Geometry: see drawing. Coordinates: mm, zero at the bounding-box minimum. A direction names the side the tool comes from. Coordinates: 2 decimals unless noted, no trailing zeros. Loops run counter-clockwise (first coordinate to the right, second up) from the corner with the lowest first, then second, coordinate; pieces in that order, holes last. Notation, with made-up numbers: M 47,83.5 L 98,83.5 A19 cw 98,104.5 Z; hole C 10,-23.5 d8. An arc over 180 degrees is marked long. One line per question, with ' | ' between items. Start each with the question number.
1. Ray query, probe 1 along Z at (x, y) = (2.5, 10); probe 2 along Y at (x, z) = (1.5, 5); probe 3 along Y at (x, z) = (8, 7.25). Return the intervals inside material, ascending.
2. Section query C-C, the plane x = 2. Output: boundary loops of the cut face in (y, z), and give its area (3 significant figures).
3. Section query A-A, the plane z = 11.5. Output: boundary loops of the cut face in (x, y), and give its area (3 significant figures).
4. Pin query (flat end, axial travel): P1, Ø1, axis at x = 7, y = 27, coming from the +Z side. Return the tip coordinate at first contact, or that it passes through.
5. Access query for the marked faces 1 and 2. Directions: +Z, -Z, +X, -X, +Y, -Y. A direction counts if a zero-diameter tool reaches every point of the face in a straight line with its end or side. Return the directions, or none.
6. Section query D-D, the plane z = 3.5. Output: boundary loops of the cut face in (x, y), and give its area (3 significant figures).
7. Mould query, pull axis Z, two halves, no side actions, for the marked faces 3, 4 and 5. Classes: pulls with the +Z half, pulls with the -Z half, needs draft (parallel to the pull), parting line crosses it, or undercut.
8. Section query B-B, the plane y = 10. Output: boundary loops of the cut face in (x, z).
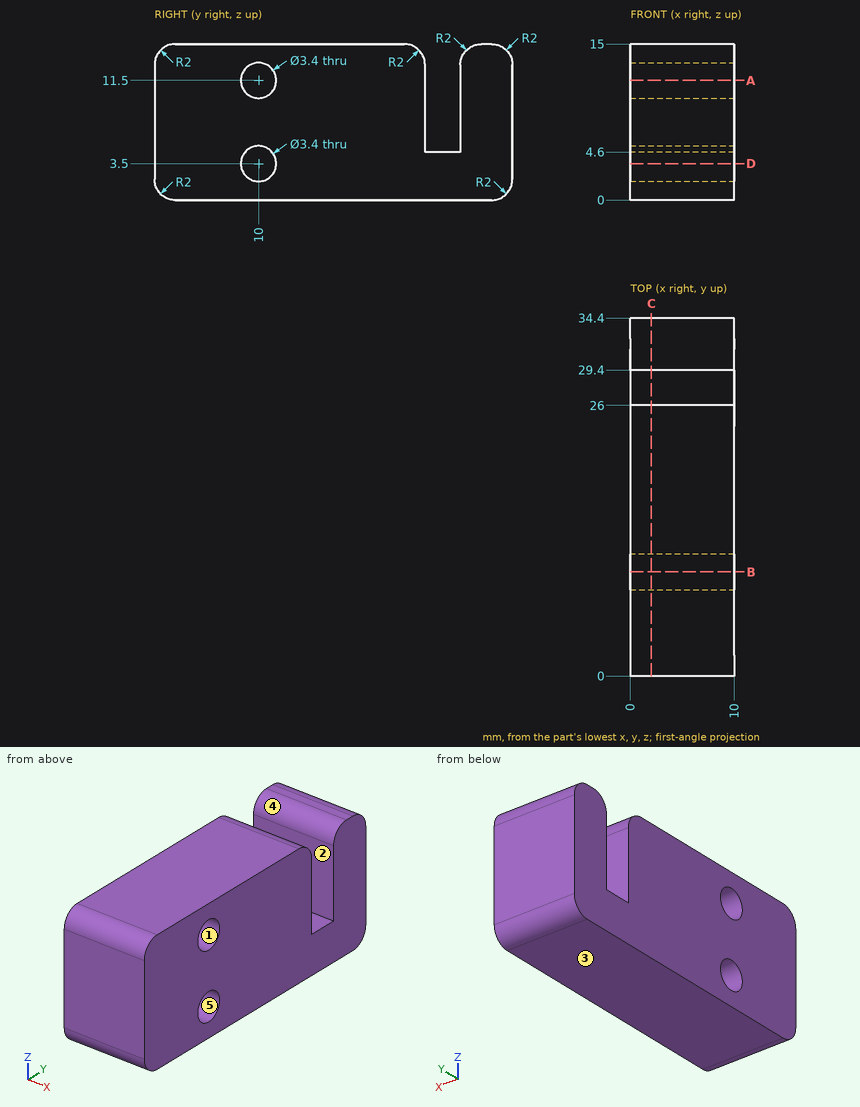
Taken from the geometry:
1) probe 1: 0 to 1.8, 5.2 to 9.8, 13.2 to 15 | probe 2: 0 to 9.2, 10.8 to 26, 29.4 to 34.4 | probe 3: 0 to 26, 29.4 to 34.4
2) outline: M 0,2 A2 ccw 2,0 L 32.4,0 A2 ccw 34.4,2 L 34.4,13 A2 ccw 32.4,15 L 31.4,15 A2 ccw 29.4,13 L 29.4,4.6 L 26,4.6 L 26,13 A2 ccw 24,15 L 2,15 A2 ccw 0,13 Z; hole C 10,3.5 d3.4; hole C 10,11.5 d3.4 | area: 457 mm^2
3) outline: M 0,0 L 10,0 L 10,8.3 L 0,8.3 Z; M 0,11.7 L 10,11.7 L 10,26 L 0,26 Z; M 0,29.4 L 10,29.4 L 10,34.4 L 0,34.4 Z | area: 276 mm^2
4) P1: z = 4.6
5) face 1: +X, -X | face 2: +Z, +X, -X
6) outline: M 0,0 L 10,0 L 10,8.3 L 0,8.3 Z; M 0,11.7 L 10,11.7 L 10,34.4 L 0,34.4 Z | area: 310 mm^2
7) face 3: pulls with the -Z half | face 4: pulls with the +Z half | face 5: undercut
8) outline: M 0,0 L 10,0 L 10,1.8 L 0,1.8 Z; M 0,5.2 L 10,5.2 L 10,9.8 L 0,9.8 Z; M 0,13.2 L 10,13.2 L 10,15 L 0,15 Z
